from build123d import *

# Parameters (mm, degrees)
SKETCH_W     = 32
SKETCH_H     = 50
SKETCH_R     = 1.75
PAD_DEPTH    = 2
SKETCH001_W  = 10
SKETCH001_H  = 12
PAD001_DEPTH = 12
SKETCH002_W  = 20
SKETCH002_H  = 8
PAD002_DEPTH = 10
SKETCH003_R  = 4
PAD003_DEPTH = 13
SKETCH004_W  = 12
SKETCH004_H  = 6
PAD004_DEPTH = 7
SKETCH005_W  = 30
SKETCH005_H  = 11.2
PAD005_DEPTH = 7.2
SKETCH006_W  = 30
SKETCH006_H  = 2.4
POCKET_DEPTH = 3.6
SKETCH007_R  = 7.2
PAD006_DEPTH = 18
FILLET_R     = 1


with BuildPart() as part:
    # Sketch → Pad (new body)
    with BuildSketch(Plane.XY):
        with Locations((16, 25)):
            Rectangle(SKETCH_W, SKETCH_H)
        with Locations((3, 47)):
            Circle(SKETCH_R, mode=Mode.SUBTRACT)
        with Locations((29, 47)):
            Circle(SKETCH_R, mode=Mode.SUBTRACT)
        with Locations((3, 3)):
            Circle(SKETCH_R, mode=Mode.SUBTRACT)
        with Locations((29, 3)):
            Circle(SKETCH_R, mode=Mode.SUBTRACT)
    extrude(amount=PAD_DEPTH)

    # Sketch001 (on Face10 of Pad) → Pad001 (join)
    with BuildSketch(Plane.XY.offset(2)):
        with Locations((16, 44)):
            Rectangle(SKETCH001_W, SKETCH001_H)
    extrude(amount=PAD001_DEPTH)

    # Sketch002 (on Face5 of Pad001) → Pad002 (join)
    with BuildSketch(Plane.XY.offset(2)):
        with Locations((16, 4)):
            Rectangle(SKETCH002_W, SKETCH002_H)
    extrude(amount=PAD002_DEPTH)

    # Sketch003 (on Face5 of Pad002) → Pad003 (join)
    with BuildSketch(Plane.XY.offset(2)):
        with Locations((27, 13)):
            Circle(SKETCH003_R)
    extrude(amount=PAD003_DEPTH)

    # Sketch004 (on Face5 of Pad003) → Pad004 (join)
    with BuildSketch(Plane.XY.offset(2)):
        with Locations((12, 13)):
            Rectangle(SKETCH004_W, SKETCH004_H)
    extrude(amount=PAD004_DEPTH)

    # Sketch005 (on Face5 of Pad004) → Pad005 (join)
    with BuildSketch(Plane.XY.offset(2)):
        with Locations((16.2, 24.6)):
            Rectangle(SKETCH005_W, SKETCH005_H)
    extrude(amount=PAD005_DEPTH)

    # Sketch006 (on Face32 of Pad005) → Pocket (cut)
    with BuildSketch(Plane.XY.offset(9.2)):
        with Locations((16.2, 21.2)):
            Rectangle(SKETCH006_W, SKETCH006_H)
        with Locations((16.2, 24.6)):
            Rectangle(SKETCH006_W, SKETCH006_H)
        with Locations((16.2, 28)):
            Rectangle(SKETCH006_W, SKETCH006_H)
    extrude(amount=-POCKET_DEPTH, mode=Mode.SUBTRACT)

    # Sketch007 (on Face6 of Pocket) → Pad006 (join)
    with BuildSketch(Plane(origin=(0, 50, 0), x_dir=(-1, 0, 0), z_dir=(0, 1, 0))):
        with Locations((-16, 8)):
            Circle(SKETCH007_R)
    extrude(amount=PAD006_DEPTH)

    # Fillet
    fillet_edges = [part.edges().sort_by_distance(p)[0] for p in [
        (23.2, 68, 8),
    ]]
    fillet(fillet_edges, radius=FILLET_R)


solid = part.part
Geometry check sheet. Reference: the model listing, model coordinates, mm. A direction names the side the tool comes from. Give positions to 0.01 mm unless a question says otherwise; leave off trailing zeros. Order: outer loops, then holes, each group sorted by start corner. A loop starts at its lowest first (then second) coordinate and runs counter-clockwise, first axis right, second up. Notation, with made-up numbers: (-26.5, 8) - (17.5, 8) arc R21 cw to (17.5, 46) - close; hole circle Ø1 at (73.25, 64). An arc over 180 degrees is marked (long way). Answer as a JSON object with one key per item and string values.
(1) Tool access check on faces 1 (the flat face through (16, 23.4, 7)), 2 (the flat face through (16.1, 50, 14.5)), 3 (the flat face through (12, 13, 9)). Record the directions out of +Z, -Z, +X, -X, +Y, -Y that give a thin tool (end or side, any length) a straight path to the whole face; none if there is none.
Report:
{"face 1": "+Z, +X, -X", "face 2": "+Z, +X, -X, -Y", "face 3": "+Z, -X"}
(2) Cross-section at A-A (x = 3). Record the cut outline in (y, z), then the cut area to 3 significant figures.
Report:
{"outline": "(0, 0) - (1.25, 0) - (1.25, 2) - (0, 2) - close; (4.75, 0) - (45.25, 0) - (45.25, 2) - (30.2, 2) - (30.2, 9.2) - (29.2, 9.2) - (29.2, 5.6) - (26.8, 5.6) - (26.8, 9.2) - (25.8, 9.2) - (25.8, 5.6) - (23.4, 5.6) - (23.4, 9.2) - (22.4, 9.2) - (22.4, 5.6) - (20, 5.6) - (20, 9.2) - (19, 9.2) - (19, 2) - (4.75, 2) - close; (48.75, 0) - (50, 0) - (50, 2) - (48.75, 2) - close", "area": "141 mm^2"}
(3) Cross-section at D-D (y = 13). Record the cut outline in (x, z), then the cut area to 3 significant figures.
Report:
{"outline": "(0, 0) - (32, 0) - (32, 2) - (31, 2) - (31, 15) - (23, 15) - (23, 2) - (18, 2) - (18, 9) - (6, 9) - (6, 2) - (0, 2) - close", "area": "252 mm^2"}
(4) Cross-section at B-B (y = 47). Record the cut outline in (x, z), then the cut area to 3 significant figures.
Report:
{"outline": "(0, 0) - (1.25, 0) - (1.25, 2) - (0, 2) - close; (4.75, 0) - (27.25, 0) - (27.25, 2) - (21, 2) - (21, 14) - (11, 14) - (11, 2) - (4.75, 2) - close; (30.75, 0) - (32, 0) - (32, 2) - (30.75, 2) - close", "area": "170 mm^2"}
(5) Depth check by flat-ended pin: pin 1 Ø4 at (y, z) = (38.5, 11) entering from +X; pin 2 Ø4 at (x, z) = (6, 2) entering from -Y; pin 3 Ø4 at (y, z) = (58.5, 4.5) entering from +X; pin 4 Ø8 at (y, z) = (47, 11.5) entering from +X. Enter the tip coordinate at first touch or a pass-through.
Report:
{"pin 1": "x = 21", "pin 2": "y = 0", "pin 3": "x = 23.04", "pin 4": "x = 23.15"}
(6) Draft check along X on faces 4 (the flat face through (18, 13, 5)), 5 (the flat face through (15.8, 50, 0.5)), 6 (the flat face through (0, 25, 1)), 7 (the flat face through (26, 4, 7)). Enter one of: released by +X, released by -X, zero draft, split by the parting line, or undercut.
Report:
{"face 4": "undercut", "face 5": "zero draft", "face 6": "released by -X", "face 7": "released by +X"}
(7) Cross-section at C-C (z = 8). State how many separate pieces and enclosed holes the cut face has, then the cut area to 3 significant figures.
Report:
{"separate pieces": "8", "enclosed holes": "0", "area": "781 mm^2"}
(8) Material ranges on line 1 (Y direction, x = 3, z = 0.6); line 2 (Y direction, x = 21.5, z = 9); line 3 (Y direction, x = 4.5, z = 7.5), recorded low to high.
Report:
{"line 1": "0 to 1.25, 4.75 to 45.25, 48.75 to 50", "line 2": "0 to 8, 19 to 20, 22.4 to 23.4, 25.8 to 26.8, 29.2 to 30.2, 50 to 68", "line 3": "19 to 20, 22.4 to 23.4, 25.8 to 26.8, 29.2 to 30.2"}
